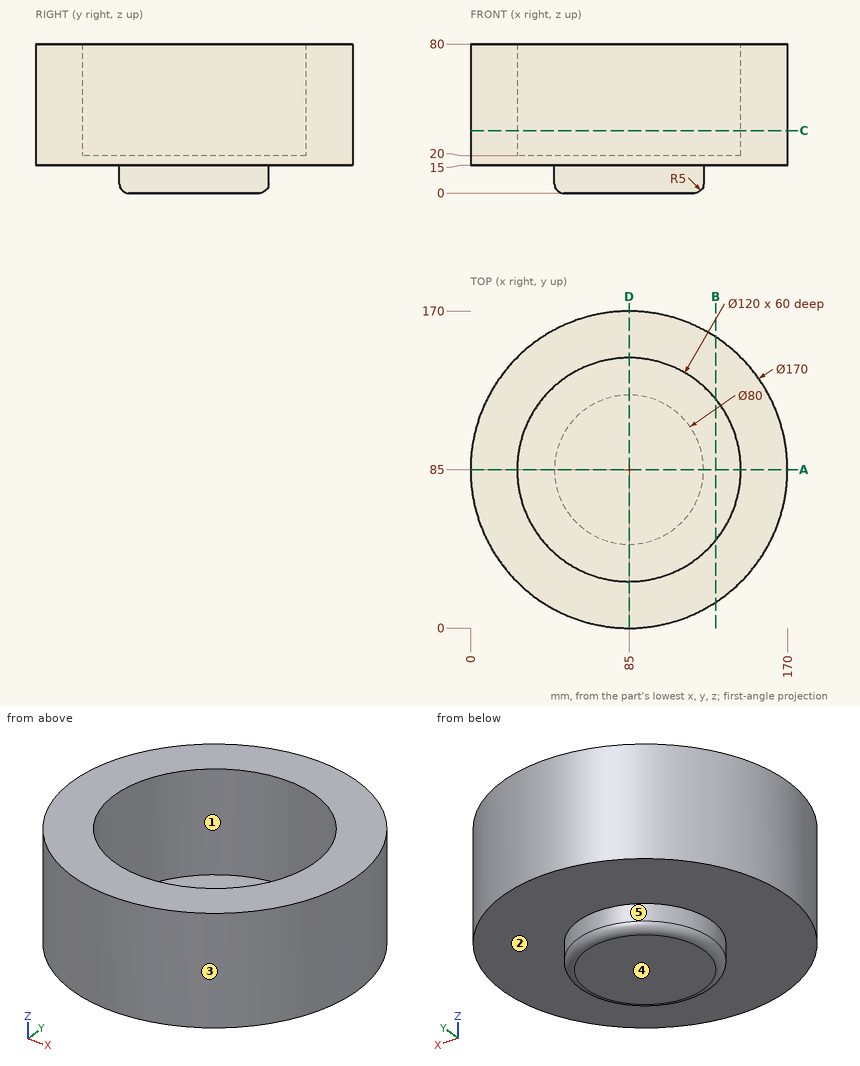
Input: dimensioned drawing with shaded views. Units: mm. Origin: part minimum x, y, z. A direction names the side the tool comes from. Round coordinates to 2 decimals unless told otherwise and drop trailing zeros. Loops run counter-clockwise (first coordinate to the right, second up) from the corner with the lowest first, then second, coordinate; pieces in that order, holes last. Notation, with made-up numbers: (79.5, 79) -> (88.5, 79) arc R25 ccw to (88.5, 92) -> close; hole circle Ø6 at (-14, -29). An arc over 180 degrees is marked (long way). Answer as a JSON object with one key per item and string values. Group by question number.
1) Section query A-A on y = 85. Output: boundary loops of the cut face in (x, z), plus the area to 3 significant figures.
2) Ray query, L1, parallel to Y at x = 85, z = 59; L2, parallel to Y at x = 113.5, z = 50; L3, parallel to Z at x = 110.5, y = 109.5. Return the intervals inside material, ascending.
3) Pin query (flat end, axial travel): pin 1 (12 mm diameter, centred on x = 126, z = 52.5, fed in from +Y); pin 2 (3 mm diameter, centred on x = 59, z = 61.5, fed in from +Y); pin 3 (3 mm diameter, centred on y = 71.5, z = 56.5, fed in from +X). Return the tip coordinate at first contact, or that it passes through.
4) Reachability of the marked faces 4 and 5 from +Z, -Z, +X, -X, +Y, -Y: full face, straight path, thin tool, end or side. Return the list, or none.
5) Section query C-C on z = 33.5. Output: boundary loops of the cut face in (x, y).
6) Section query B-B on x = 131.5. Output: boundary loops of the cut face in (y, z).
7) Draft query along X for the marked faces 1, 2 and 3. Return one class per face: +X half, -X half, draft (parallel to the pull), parting line (faces both ways), or undercut.
Reply:
{
 "1": {"outline": "(0, 15) -> (45, 15) -> (45, 5) arc R5 ccw to (50, 0) -> (120, 0) arc R5 ccw to (125, 5) -> (125, 15) -> (170, 15) -> (170, 80) -> (145, 80) -> (145, 20) -> (25, 20) -> (25, 80) -> (0, 80) -> close", "area": "5,040 mm2"},
 "2": {"L1": "y = 0 to 25, 145 to 170", "L2": "y = 4.92 to 32.2, 137.8 to 165.08", "L3": "z = 0.01 to 20"},
 "3": {"pin 1": "stops at y = 162.46", "pin 2": "stops at y = 166.39", "pin 3": "stops at x = 169.15"},
 "4": {"face 4": "-Z, +X, -X, +Y, -Y", "face 5": "-Z"},
 "5": {"outline": "circle Ø170 at (85, 85); hole circle Ø120 at (85, 85)"},
 "6": {"outline": "(13.85, 15) -> (156.15, 15) -> (156.15, 80) -> (122.92, 80) -> (122.92, 20) -> (47.08, 20) -> (47.08, 80) -> (13.85, 80) -> close"},
 "7": {"face 1": "undercut", "face 2": "draft", "face 3": "parting line"}
}
